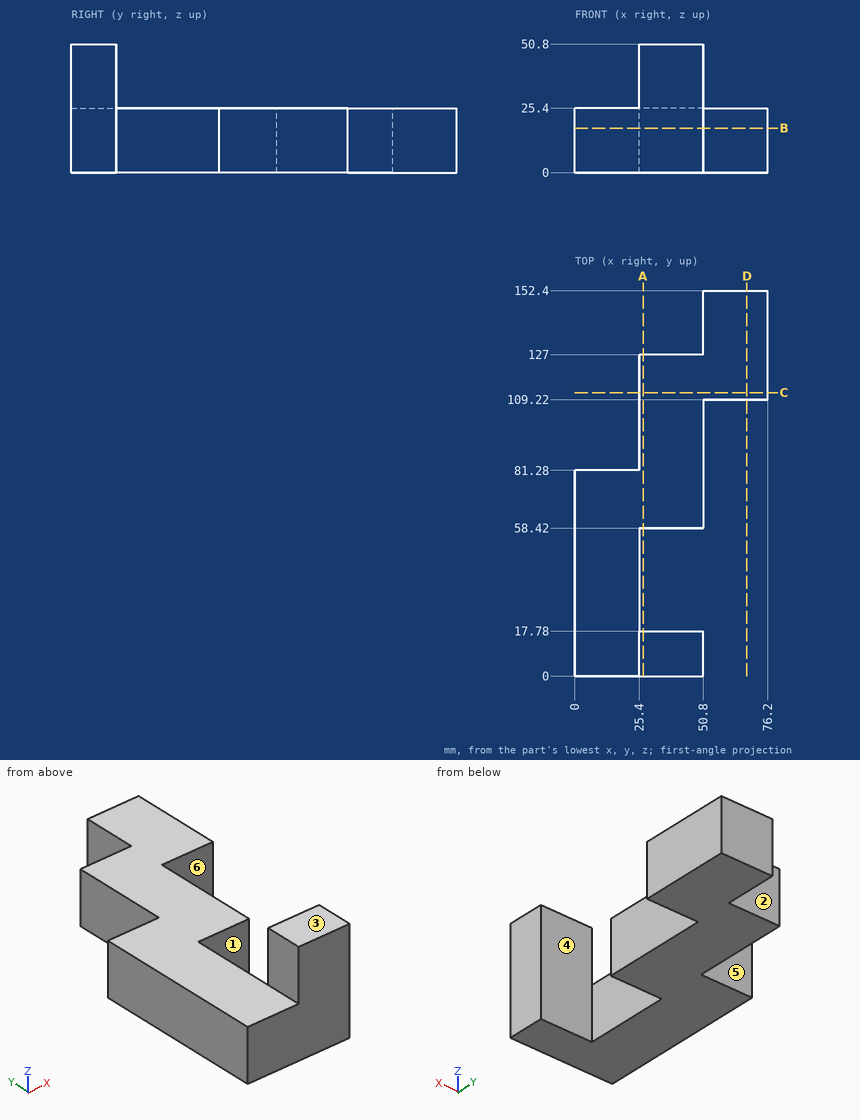
Answer from the drawing. Dimensions are ordinates in mm from the lowest x, y and z of the part. A direction names the side the tool comes from. Coordinates: 2 decimals unless noted, no trailing zeros. Order: outer loops, then holes, each group sorted by start corner. A loop starts at its lowest first (then second) coordinate and runs counter-clockwise, first axis right, second up. Notation, with made-up numbers: M -34,2 L -15,2 A16 ccw -15,26 Z; hole C 74,81 d6. An arc over 180 degrees is marked long. Put each result on its own line as item: value. Start each with the question number.
Item 1: Given pin 1 Ø20.5 at (y, z) = (48, 17) entering from +X; pin 2 Ø20.5 at (x, z) = (12.5, 7.5) entering from +Y; pin 3 Ø9 at (y, z) = (13, 34) entering from +X, each flat-ended and moving along its own axis, determine where each tip first touches the part or whether it passes through.
Item 2: Section B-B, the plane z = 17.5 is taken. Determine the outline of the cut face in (x, y).
Item 3: The mould has two halves that part along Y. Classify the marked faces 1, 2 and 3: +Y half, -Y half, draft (parallel to the pull), parting line (faces both ways), or undercut.
Item 4: Section A-A, the plane x = 27 is taken. Determine the outline of the cut face in (y, z), plus the area to 3 significant figures.
Item 5: Consider probe 1 along Y at (x, z) = (49.5, 11); probe 2 along Y at (x, z) = (52, 10.5); probe 3 along Z at (x, y) = (33, 72.5). Determine where each line is inside the solid, lowest interval first. Write a range as [from, to].
Item 6: Section D-D, the plane x = 68 is taken. Determine the outline of the cut face in (y, z).
Item 7: Section C-C, the plane y = 112 is taken. Determine the outline of the cut face in (x, z), plus the area to 3 significant figures.
Item 8: For the marked faces 4, 5 and 6, determine the directions among +Z, -Z, +X, -X, +Y, -Y from which every point of the face is accessible in a straight line to the end or side of a thin tool.
Computed:
1. pin 1: stops at x = 25.4
1. pin 2: stops at y = 81.28
1. pin 3: stops at x = 50.8
2. outline: M 0,0 L 50.8,0 L 50.8,17.78 L 25.4,17.78 L 25.4,58.42 L 50.8,58.42 L 50.8,109.22 L 76.2,109.22 L 76.2,152.4 L 50.8,152.4 L 50.8,127 L 25.4,127 L 25.4,81.28 L 0,81.28 Z
3. face 1: undercut
3. face 2: +Y half
3. face 3: draft
4. outline: M 0,0 L 17.78,0 L 17.78,50.8 L 0,50.8 Z; M 58.42,0 L 127,0 L 127,25.4 L 58.42,25.4 Z
4. area: 2,650 mm2
5. probe 1: y = [0, 17.78], [58.42, 127]
5. probe 2: y = [109.22, 152.4]
5. probe 3: z = [0, 25.4]
6. outline: M 109.22,0 L 152.4,0 L 152.4,25.4 L 109.22,25.4 Z
7. outline: M 25.4,0 L 76.2,0 L 76.2,25.4 L 25.4,25.4 Z
7. area: 1,290 mm2
8. face 4: +Z, -Z, +X
8. face 5: +Z, -Z, -X, +Y
8. face 6: +Z, -Z, +X, -Y
